```python
from build123d import *

# Parameters (mm, degrees)
BOSS_EXTRUDE2_DEPTH = 10
SKETCH5_R           = 0.635
CUT_EXTRUDE1_DEPTH  = 10
CUT_EXTRUDE1_DRAFT  = 1.2


with BuildPart() as part:
    # Sketch2 → Boss-Extrude2 (new body)
    with BuildSketch(Plane(origin=(0, 0, 0), x_dir=(1, 0, 0), z_dir=(0, 1, 0))):
        with BuildLine():
            Line((0.055343897, 0.632583633), (0.075113859, 0.858555332))
            ThreePointArc((0.075113859, 0.858555332), (0.329887136, 1.190582332), (0.738477631, 1.1))
            Line((0.738477631, 1.1), (1.382842712, 0.455634919))
            ThreePointArc((1.382842712, 0.455634919), (1.665996883, 0.266437351), (2, 0.2))
            Line((2, 0.2), (4.2, 0.2))
            ThreePointArc((4.2, 0.2), (4, 0), (4.2, -0.2))
            Line((4.2, -0.2), (2, -0.2))
            ThreePointArc((2, -0.2), (1.665996883, -0.266437351), (1.382842712, -0.455634919))
            Line((1.382842712, -0.455634919), (0.738477631, -1.1))
            ThreePointArc((0.738477631, -1.1), (0.329887136, -1.190582332), (0.075113859, -0.858555332))
            Line((0.075113859, -0.858555332), (0.055343897, -0.632583633))
            Line((0.055343897, -0.632583633), (0.055343897, 0.632583633))
        make_face()
    extrude(amount=BOSS_EXTRUDE2_DEPTH)


with BuildPart() as cut_extrude1_tool:
    # Sketch5 → Cut-Extrude1 (with draft: the straight prism first)
    with BuildSketch(Plane.XZ):
        Circle(SKETCH5_R)
    extrude(amount=-CUT_EXTRUDE1_DEPTH)
    # Cut-Extrude1: the draft: its side faces are tilted about the plane it starts from
    cut_extrude1_sides = [cut_extrude1_tool.faces().sort_by_distance(p)[0] for p in [
        (-0.635, 5, 0),
    ]]
    draft(cut_extrude1_sides, Plane.XZ, CUT_EXTRUDE1_DRAFT)


with BuildPart() as part_1:
    add(part.part)

    # Cut-Extrude1: cut by cut_extrude1_tool
    add(cut_extrude1_tool.part, mode=Mode.SUBTRACT)


solid = part_1.part
```
Part model, mm, in its own coordinate system. A direction names the side the tool comes from. Coordinates: 2 decimals unless noted, no trailing zeros. Write each loop counter-clockwise with the first axis right and the second up, starting at its lowest first coordinate (ties: lowest second). Pieces come first, ordered by that corner, then holes.
Item 1: Probe line 1 (Z direction, x = 3.1, y = 1.5); line 2 (Z direction, x = 1, y = 0.5); line 3 (Z direction, x = 0.7, y = 7). List the from-to ranges inside material, lowest first.
Item 2: Slice it at A-A (y = 4). Write the cut outline in (x, z).
Item 3: Slice it at C-C (y = 1). Write the cut outline in (x, z).
Item 4: Slice it at B-B (x = 3.4). Write the cut outline in (y, z).
Item 5: Slice it at D-D (z = 0). Write the cut outline in (x, y) (3 decimals).
Item 6: Pin check, flat tips, straight feed: pin 1 (1.8 mm diameter, centred on x = 3.5, y = 3.5, fed in from -Z); pin 2 (1 mm diameter, centred on x = 2.5, z = -0.5, fed in from -Y); pin 3 (1.1 mm diameter, centred on x = 2.5, y = 4.5, fed in from +Z). Stop position of each tip, or through.
Item 7: Which spindle directions (+Z, -Z, +X, -X, +Y, -Y) get a long thin tool onto all of the face, cutting with end or side? Do faces 1 (the face through (0.738, 4.93, -0.015)), 2 (the face through (3, 5, 0.2)), 3 (the face through (2, 10, 0)), 4 (the face through (3, 5, -0.2)). Say none if no direction does.
Results found:
1. line 1: z = -0.2 to 0.2
1. line 2: z = -0.84 to 0.84
1. line 3: z = -1.13 to -0.35, 0.35 to 1.13
2. outline: (0.06, -0.72) - (0.08, -0.86) arc R0.39 ccw to (0.74, -1.1) - (1.38, -0.46) arc R0.87 cw to (2, -0.2) - (4.2, -0.2) arc R0.2 cw to (4.2, 0.2) - (2, 0.2) arc R0.87 cw to (1.38, 0.46) - (0.74, 1.1) arc R0.39 ccw to (0.08, 0.86) - (0.06, 0.72) arc R0.72 cw to start
3. outline: (0.06, -0.65) - (0.08, -0.86) arc R0.39 ccw to (0.74, -1.1) - (1.38, -0.46) arc R0.87 cw to (2, -0.2) - (4.2, -0.2) arc R0.2 cw to (4.2, 0.2) - (2, 0.2) arc R0.87 cw to (1.38, 0.46) - (0.74, 1.1) arc R0.39 ccw to (0.08, 0.86) - (0.06, 0.65) arc R0.66 cw to start
4. outline: (0, -0.2) - (10, -0.2) - (10, 0.2) - (0, 0.2) - close
5. outline: (0.635, 0) - (4, 0) - (4, 10) - (0.844, 10) - close
6. pin 1: stops at z = -0.2
6. pin 2: stops at y = 0
6. pin 3: stops at z = 0.2
7. face 1: -X, +Y
7. face 2: +Z, +X, +Y, -Y
7. face 3: +Z, -Z, +X, -X, +Y
7. face 4: -Z, +X, +Y, -Y
